Geometry: final body of the model. Coordinates: model frame, mm. A direction names the side the tool comes from. Coordinates: 2 decimals unless noted, no trailing zeros. Write each loop counter-clockwise with the first axis right and the second up, starting at its lowest first coordinate (ties: lowest second). Pieces come first, ordered by that corner, then holes.
from build123d import *

# Parameters (mm, degrees)
F1_DEPTH = 100
F2_R     = 3.5
F3_DEPTH = 100


with BuildPart() as f1:
    # F0 (on Front) → F1 (new body)
    with BuildSketch(Plane.XZ):
        Polygon((5.189254, 40), (5.189254, 0), (5.189254, -40), (30.189254, -40), (30.189254, -8), (55.189254, -8), (55.189254, 8), (30.189254, 8), (30.189254, 40), align=None)
    extrude(amount=F1_DEPTH)

    # F2 (on face) → F3 (cut)
    with BuildSketch(Plane(origin=(5.189254, 0, 0), x_dir=(0, -1, 0), z_dir=(-1, 0, 0))):
        with Locations((25, 30)):
            Circle(F2_R)
        with Locations((75, 30)):
            Circle(F2_R)
        with Locations((25, -30)):
            Circle(F2_R)
        with Locations((75, -30)):
            Circle(F2_R)
    extrude(amount=-F3_DEPTH, mode=Mode.SUBTRACT)


solid = f1.part
Item 1: Section C-C, the plane z = -30. Output: boundary loops of the cut face in (x, y), plus the area to 3 significant figures.
Derived:
outline: (5.19, -100) - (30.19, -100) - (30.19, -78.5) - (5.19, -78.5) - close; (5.19, -71.5) - (30.19, -71.5) - (30.19, -28.5) - (5.19, -28.5) - close; (5.19, -21.5) - (30.19, -21.5) - (30.19, 0) - (5.19, 0) - close
area: 2,150 mm2
Item 2: Pull-direction query (Y, two-part tool) for faces 4 (the cylindrical face through (17.51, -24.54, 33.47)), 5 (the flat face through (19, 0, 1)), 6 (the flat face through (18, -49, 40)); classes: released by +Y, released by -Y, zero draft, split by the parting line, or undercut.
Derived:
face 4: undercut
face 5: released by +Y
face 6: zero draft
Item 3: Section D-D, the plane y = -49.5. Output: boundary loops of the cut face in (x, z).
Derived:
outline: (5.19, -40) - (30.19, -40) - (30.19, -8) - (55.19, -8) - (55.19, 8) - (30.19, 8) - (30.19, 40) - (5.19, 40) - close
Item 4: Section A-A, the plane y = -75. Output: boundary loops of the cut face in (x, z), plus the area to 3 significant figures.
Derived:
outline: (5.19, -40) - (30.19, -40) - (30.19, -33.5) - (5.19, -33.5) - close; (5.19, -26.5) - (30.19, -26.5) - (30.19, -8) - (55.19, -8) - (55.19, 8) - (30.19, 8) - (30.19, 26.5) - (5.19, 26.5) - close; (5.19, 33.5) - (30.19, 33.5) - (30.19, 40) - (5.19, 40) - close
area: 2,050 mm2
Item 5: Pin query (flat end, axial travel): pin 1 (7.5 mm diameter, centred on x = 39, y = -70.5, fed in from +Z); pin 2 (6.5 mm diameter, centred on y = -75, z = -30, fed in from +X); pin 3 (20 mm diameter, centred on x = 43.5, y = -54.5, fed in from -Z); pin 4 (16 mm diameter, centred on y = -40, z = -17, fed in from +X). Return the tip coordinate at first contact, or that it passes through.
Derived:
pin 1: stops at z = 8
pin 2: passes through
pin 3: stops at z = -8
pin 4: stops at x = 30.19
Item 6: Section B-B, the plane x = 18. Output: boundary loops of the cut face in (y, z).
Derived:
outline: (-100, -40) - (0, -40) - (0, 40) - (-100, 40) - close; hole circle Ø7 at (-75, -30); hole circle Ø7 at (-75, 30); hole circle Ø7 at (-25, -30); hole circle Ø7 at (-25, 30)
Item 7: Material intervals for probe 1 along Z at (x, y) = (11, -75); probe 2 along Y at (x, z) = (21.5, 31.5); probe 3 along X at (y, z) = (-39, 23.5), sorted ascending.
Derived:
probe 1: z = -40 to -33.5, -26.5 to 26.5, 33.5 to 40
probe 2: y = -100 to -78.16, -71.84 to -28.16, -21.84 to 0
probe 3: x = 5.19 to 30.19
Item 8: Set-up query: faces 1 (the flat face through (43, -49, -8)), 2 (the flat face through (30.189, -49, 24)), 3 (the flat face through (19, -100, 1)). Return all of +Z, -Z, +X, -X, +Y, -Y with unobstructed straight access to the full face (end or side cutting, diameter ignored); none if empty.
Derived:
face 1: -Z, +X, +Y, -Y
face 2: +Z, +X, +Y, -Y
face 3: +Z, -Z, +X, -X, -Y
